```python
from build123d import *

# Parameters (mm, degrees)
SKETCH3_R           = 1.1
BOSS_EXTRUDE1_DEPTH = 7.5
SHELL1_START        = 0.5
SHELL1_OUTLINE_R    = 1.6
SHELL1_DEPTH        = 6.5
SKETCH5_W           = 36.304347826
SKETCH5_H           = 6.5
BOSS_EXTRUDE2_DEPTH = 1
CUT_EXTRUDE2_DEPTH  = 24.369518609
SKETCH7_R           = 1.1
CUT_EXTRUDE3_DEPTH  = 24.524123788
SKETCH10_W          = 87.275560702
SKETCH10_H          = 0.8
CUT_EXTRUDE15_DEPTH = 0.499
SKETCH11_R          = 1.1
CUT_EXTRUDE16_DEPTH = 24.805553974


# Read off the part's stored shape, not the designer's step: Shell1
with BuildPart() as part:
    # Sketch3 → Boss-Extrude1 (new body)
    with BuildSketch(Plane(origin=(0, 0, 0), x_dir=(1, 0, 0), z_dir=(0, 1, 0))):
        with BuildLine():
            Line((-15.88, 2.8), (6.52, 2.8))
            Line((6.52, 2.8), (22.12, -1.8))
            Line((22.12, -1.8), (-15.88, -1.8))
            ThreePointArc((-15.88, -1.8), (-18.18, 0.5), (-15.88, 2.8))
        make_face()
        with Locations(Location((-15.88, 0.5, 0), (0, 0, 270))):
            Circle(SKETCH3_R, mode=Mode.SUBTRACT)
    extrude(amount=BOSS_EXTRUDE1_DEPTH)

    # Shell1 outline → Shell1 (cut)
    with BuildSketch(Plane(origin=(0, 0, 0), x_dir=(1, 0, 0), z_dir=(0, 1, 0)).offset(SHELL1_START)):
        with BuildLine():
            Line((6.52, 2.8), (-15.88, 2.8))
            Line((-15.88, 2.8), (-15.88, 2.3))
            ThreePointArc((-15.88, 2.3), (-17.68, 0.5), (-15.88, -1.3))
            Line((-15.88, -1.3), (20.424347826, -1.3))
            Line((20.424347826, -1.3), (6.52, 2.8))
        make_face()
        with Locations((-15.88, 0.5)):
            Circle(SHELL1_OUTLINE_R, mode=Mode.SUBTRACT)
    extrude(amount=SHELL1_DEPTH, mode=Mode.SUBTRACT)

    # Sketch5 → Boss-Extrude2 (add)
    with BuildSketch(Plane(origin=(0, 0, 1.3), x_dir=(-1, 0, 0), z_dir=(0, 0, -1))):
        with Locations((-2.272173913, 3.75)):
            Rectangle(SKETCH5_W, SKETCH5_H)
    extrude(amount=BOSS_EXTRUDE2_DEPTH)

    # Sketch6 → Cut-Extrude2 (cut, through all)
    with BuildSketch(Plane(origin=(0, 7, 0), x_dir=(1, 0, 0), z_dir=(0, 1, 0))):
        Polygon((20.424347826, -0.3), (17.033043478, -0.3), (20.424347826, -1.3), align=None)
    extrude(amount=-CUT_EXTRUDE2_DEPTH, mode=Mode.SUBTRACT)

    # Sketch7 → Cut-Extrude3 (cut, through all)
    with BuildSketch(Plane(origin=(0, 7.5, 0), x_dir=(1, 0, 0), z_dir=(0, 1, 0))):
        with Locations(Location((-15.88, 0.5, 0), (0, 0, 270))):
            Circle(SKETCH7_R)
    extrude(amount=-CUT_EXTRUDE3_DEPTH, mode=Mode.SUBTRACT)

    # Sketch10 → Cut-Extrude15 (cut)
    with BuildSketch(Plane.XY.offset(1.8)):
        with Locations((23.190230884, 6.1)):
            Rectangle(SKETCH10_W, SKETCH10_H)
    extrude(amount=-CUT_EXTRUDE15_DEPTH, mode=Mode.SUBTRACT)

    # Sketch11 → Cut-Extrude16 (cut, through all)
    with BuildSketch(Plane.XY.offset(1.8)):
        with Locations((-6.23, 3.2)):
            Circle(SKETCH11_R)
        with Locations((10.1714, 3.2)):
            Circle(SKETCH11_R)
    extrude(amount=-CUT_EXTRUDE16_DEPTH, mode=Mode.SUBTRACT)


solid = part.part
```
The model under review builds one solid part; all positions refer to its coordinate system, in mm. A direction names the side the tool comes from. Coordinates: 2 decimals unless noted, no trailing zeros. Write each loop counter-clockwise with the first axis right and the second up, starting at its lowest first coordinate (ties: lowest second). Pieces come first, ordered by that corner, then holes. Notation, with made-up numbers: (43, -38) - (77, -38) arc R17 cw to (77, -10) - close; hole circle Ø6 at (1, 83). An arc over 180 degrees is marked (long way). Answer in a Markdown table with one row per item. Add a question column.
Q1. Consider section B-B on y = 3.2. Give the boundary of the cut face in (x, z).
Q2. Clearance check with flat-ended pins moving along their axes: pin 1 (2 mm diameter, centred on y = 3, z = 1, fed in from -X) (3 decimals); pin 2 (1.8 mm diameter, centred on x = -15.88, z = -0.5, fed in from -Y); pin 3 (2 mm diameter, centred on x = 7, z = 0, fed in from -Y). State where each tip first meets the part, or that it passes through.
Q3. To check wall thickness, follow line 1 along X through (y, z) = (4, -0.8); line 2 along Y through (x, z) = (1, -2.35); line 3 along X through (y, z) = (4.5, -0.9) (3 decimals). State the ranges of each line that lie inside material, in increasing order. Write a range as from..to.
Q4. Consider section C-C on y = 5.25. Give the boundary of the cut face in (x, z), then the cut area to 3 significant figures.
Q5. Draft analysis for pull direction Z (two halves, no side actions). For faces 1 (the face through (-16.856, 3.698, 0.008)), 2 (the face through (1, 6, 1.301)), 3 (the face through (11.19, 2.78, 1.06)), state which applies: +Z half, -Z half, draft (parallel to the pull), parting line (faces both ways), or undercut.
Q6. Consider section D-D on x = -6.23. Give the boundary of the cut face in (y, z), then the cut area to 3 significant figures.
Q7. For faces 4 (the face through (-16.629, 3.704, -1.914)), 5 (the face through (3, 7, 1.8)), list the 3-axis set-ups (+Z, -Z, +X, -X, +Y, -Y) from which the entire face can be reached by the end or side of a thin tool; tool diameter is ignored.
Q8. Consider section A-A on z = -0.5. Give the boundary of the cut face in (x, y).
Answers below:
| question | item | result |
|---|---|---|
| 1 | outline | (-15.88, -2.8) - (-15.88, -2.3) arc R1.8 cw to (-15.88, 1.3) - (-15.88, 1.1) arc R1.6 ccw (long way) to (-14.49, 0.3) - (-7.33, 0.3) - (-7.33, 1.8) - (-15.88, 1.8) arc R2.3 ccw to start; (-5.13, 0.3) - (9.07, 0.3) - (9.07, 1.8) - (-5.13, 1.8) - close; (11.27, 0.3) - (17.03, 0.3) - (22.12, 1.8) - (11.27, 1.8) - close; hole circle Ø2.2 at (-15.88, -0.5) |
| 2 | pin 1 | x = -18.125 |
| 2 | pin 2 | through |
| 2 | pin 3 | y = 0 |
| 3 | line 1 | -18.16..-17.65, -17.45..-16.94, -14.82..-14.31 |
| 3 | line 2 | 0..0.5, 7..7.5 |
| 3 | line 3 | -18.145..-17.635, -17.429..-16.905, -14.855..-14.331 |
| 4 | outline | (-15.88, -2.8) - (-15.88, -2.3) arc R1.8 cw to (-15.88, 1.3) - (-15.88, 1.1) arc R1.6 ccw (long way) to (-14.49, 0.3) - (17.03, 0.3) - (22.12, 1.8) - (-15.88, 1.8) arc R2.3 ccw to start; hole circle Ø2.2 at (-15.88, -0.5) |
| 4 | area | 59.9 mm² |
| 5 | face 1 | undercut |
| 5 | face 2 | +Z half |
| 5 | face 3 | draft |
| 6 | outline | (0, -2.8) - (0.5, -2.8) - (0.5, 0.3) - (2.1, 0.3) - (2.1, 1.8) - (0, 1.8) - close; (4.3, 0.3) - (7, 0.3) - (7, -2.8) - (7.5, -2.8) - (7.5, 1.8) - (6.5, 1.8) - (6.5, 1.3) - (5.7, 1.3) - (5.7, 1.8) - (4.3, 1.8) - close |
| 6 | area | 10.7 mm² |
| 7 | face 4 | none |
| 7 | face 5 | +Z, +X, -X, +Y, -Y |
| 8 | outline | (-18.18, 0) - (-16.98, 0) - (-16.98, 7.5) - (-18.18, 7.5) - close; (-14.78, 0) - (14.32, 0) - (14.32, 0.5) - (-14.28, 0.5) - (-14.28, 7) - (14.32, 7) - (14.32, 7.5) - (-14.78, 7.5) - close; hole (-17.68, 0.5) - (-17.48, 0.5) - (-17.48, 7) - (-17.68, 7) - close |
